Read the model definition and answer for the solid it produces. Units are mm, in the model's axes. A direction names the side the tool comes from. Give positions to 0.01 mm unless a question says otherwise; leave off trailing zeros. Order: outer loops, then holes, each group sorted by start corner. A loop starts at its lowest first (then second) coordinate and runs counter-clockwise, first axis right, second up. Notation, with made-up numbers: M 41,-18.5 L 96,-18.5 A26 ccw 96,-0.5 Z; hole C 86,66.25 d2. An arc over 180 degrees is marked long. Write item = value, one per line. Start each with the question number.
from build123d import *

# Parameters (mm, degrees)
F0_R     = 1.5
F0_W     = 1.8
F0_H     = 10
F1_DEPTH = 3


with BuildPart() as f1:
    # F0 (on Right) → F1 (new body)
    with BuildSketch(Plane.YZ):
        with BuildLine():
            Line((-27, 20.833333), (-30, 20.833333))
            Line((-30, 20.833333), (-30, -20.833333))
            Line((-30, -20.833333), (-27, -20.833333))
            Line((-27, -20.833333), (-27, -62.5))
            Line((-27, -62.5), (-18, -62.5))
            Line((-18, -62.5), (-9, -62.5))
            Line((-9, -62.5), (-9, -59.5))
            Line((-9, -59.5), (0, -59.5))
            Line((0, -59.5), (0, -53.7))
            ThreePointArc((0, -53.7), (-1.5, -52.2), (0, -50.7))
            Line((0, -50.7), (0, 50.7))
            ThreePointArc((0, 50.7), (-1.5, 52.2), (0, 53.7))
            Line((0, 53.7), (0, 59.5))
            Line((0, 59.5), (-9, 59.5))
            Line((-9, 59.5), (-9, 62.5))
            Line((-9, 62.5), (-18, 62.5))
            Line((-18, 62.5), (-27, 62.5))
            Line((-27, 62.5), (-27, 20.833333))
        make_face()
        with Locations((-19.7, 0)):
            Circle(F0_R, mode=Mode.SUBTRACT)
        with Locations((-12.4, 0)):
            Rectangle(F0_W, F0_H, mode=Mode.SUBTRACT)
        with BuildLine():
            Line((9, 59.5), (0, 59.5))
            Line((0, 59.5), (0, 53.7))
            ThreePointArc((0, 53.7), (1.5, 52.2), (0, 50.7))
            Line((0, 50.7), (0, -50.7))
            ThreePointArc((0, -50.7), (1.5, -52.2), (0, -53.7))
            Line((0, -53.7), (0, -59.5))
            Line((0, -59.5), (9, -59.5))
            Line((9, -59.5), (9, -62.5))
            Line((9, -62.5), (18, -62.5))
            Line((18, -62.5), (27, -62.5))
            Line((27, -62.5), (27, -20.833333))
            Line((27, -20.833333), (30, -20.833333))
            Line((30, -20.833333), (30, 20.833333))
            Line((30, 20.833333), (27, 20.833333))
            Line((27, 20.833333), (27, 62.5))
            Line((27, 62.5), (18, 62.5))
            Line((18, 62.5), (9, 62.5))
            Line((9, 62.5), (9, 59.5))
        make_face()
        with Locations((12.4, 0)):
            Rectangle(F0_W, F0_H, mode=Mode.SUBTRACT)
        with Locations((19.7, 0)):
            Circle(F0_R, mode=Mode.SUBTRACT)
    extrude(amount=F1_DEPTH)


solid = f1.part
1) Find the intervals of material crossed by probe 1 along Y at (x, z) = (1, -52.2); probe 2 along Z at (x, y) = (2.3, -19.7); probe 3 along Y at (x, z) = (2.45, 26), in increasing order. Write a range as [from, to].
2) For a pull along Z with two mould halves and no side action, classify faces 6 (the face through (1.5, -0.9, 51)), 7 (the face through (1, 29, 20.833)), 8 (the face through (1, 30, 0)) as pulls with the +Z half, pulls with the -Z half, needs draft (parallel to the pull), parting line crosses it, or undercut.
3) Each of these flat-tipped pins is pushed along its axis until it touches: P1, Ø1, axis at x = 1.5, z = 40, coming from the -Y side; P2, Ø0.9, axis at x = 1.5, y = -29, coming from the -Z side; P3, Ø1.5, axis at x = 1, y = 29, coming from the +Z side. Where does it stop, or does it pass through?
4) For faces 1 (the face through (1, -27, 42)), 2 (the face through (1, 27, 41)), 3 (the face through (1, -9, -61)), 4 (the face through (1, -11.5, 0)), 5 (the face through (1, -27, -41)), determine the directions among +Z, -Z, +X, -X, +Y, -Y from which every point of the face is accessible in a straight line to the end or side of a thin tool.
5) Find section D-D on y = 19.7. Determine the outline of the cut face in (x, z).
6) Find section B-B on x = 1.85. Count the separate pieces of the cut face and the enclosed holes in it, plus the area to 3 significant figures.
7) Find section A-A on y = 0. Determine the outline of the cut face in (x, z), plus the area to 3 significant figures.
8) Find section C-C on z = 0. Determine the outline of the cut face in (x, y), plus the area to 3 significant figures.
Numbers:
q1.probe_1 = [-27, -1.5], [1.5, 27]
q1.probe_2 = [-62.5, -1.5], [1.5, 62.5]
q1.probe_3 = [-27, 27]
q2.face_6 = undercut
q2.face_7 = pulls with the +Z half
q2.face_8 = needs draft
q3.P1 = -27
q3.P2 = -20.83
q3.P3 = 20.83
q4.face_1 = +Z, +X, -X, -Y
q4.face_2 = +Z, +X, -X, +Y
q4.face_3 = -Z, +X, -X
q4.face_4 = +X, -X
q4.face_5 = -Z, +X, -X, -Y
q5.outline = M 0,-62.5 L 3,-62.5 L 3,-1.5 L 0,-1.5 Z; M 0,1.5 L 3,1.5 L 3,62.5 L 0,62.5 Z
q6.separate_pieces = 1
q6.enclosed_holes = 6
q6.area = 6,830 mm2
q7.outline = M 0,-59.5 L 3,-59.5 L 3,-53.7 L 0,-53.7 Z; M 0,-50.7 L 3,-50.7 L 3,50.7 L 0,50.7 Z; M 0,53.7 L 3,53.7 L 3,59.5 L 0,59.5 Z
q7.area = 339 mm2
q8.outline = M 0,-30 L 3,-30 L 3,-21.2 L 0,-21.2 Z; M 0,-18.2 L 3,-18.2 L 3,-13.3 L 0,-13.3 Z; M 0,-11.5 L 3,-11.5 L 3,11.5 L 0,11.5 Z; M 0,13.3 L 3,13.3 L 3,18.2 L 0,18.2 Z; M 0,21.2 L 3,21.2 L 3,30 L 0,30 Z
q8.area = 151 mm2
